Design review of the part built by this model. Coordinates are the model's own, in mm. Give positions to 0.01 mm unless a question says otherwise; leave off trailing zeros. Loops run counter-clockwise (first coordinate to the right, second up) from the corner with the lowest first, then second, coordinate; pieces in that order, holes last. Notation, with made-up numbers: M -19.75,-36.5 L 25.25,-36.5 A20 cw 25.25,-27.5 Z; hole C -30.5,83.25 d4. An arc over 180 degrees is marked long. Use a Markdown table: item, result. Add a question column.
(1) For probe 1 along Y at (x, z) = (40, 3.25); probe 2 along Y at (x, z) = (-7.75, 4.75); probe 3 along X at (y, z) = (13.5, 9), list the stretches that pass through material, from the lowest coordinate up.
(2) Add section A-A, the plane x = -40. Give the boundary of the cut face in (y, z).
(3) Insertion check: pin 1 Ø2.5 at (x, y) = (15.5, 0) entering from +Z. The pin has a flat end and moves straight along its axis. Give the tip position at first contact, or say it passes through.
(4) Draft analysis for pull direction Y (two halves, no side actions). For faces 1 (the face through (-43, 33, 6)), 2 (the face through (-1, 43, 6)), 3 (the face through (-1, -57, 6)), state which applies: pulls with the +Y half, pulls with the -Y half, needs draft (parallel to the pull), parting line crosses it, or undercut.
(5) Add section C-C, the plane x = -7.75. Give the boundary of the cut face in (y, z).
(6) Add section B-B, the plane y = -7. Give the boundary of the cut face in (x, z).
(7) Add section D-D, the plane z = 10. State how many separate pieces and enclosed holes the cut face has, then the cut area to 3 significant figures.
```python
from build123d import *

# Parameters (mm, degrees)
ESQUISSE1_R             = 18.5
BOSS_EXTRU_1_DEPTH      = 12
ESQUISSE2_R             = 2
ENL_V_MAT_EXTRU_1_DEPTH = 13
ESQUISSE3_R             = 6.25
ENL_V_MAT_EXTRU_2_DEPTH = 13
ESQUISSE4_W             = 100
ESQUISSE4_H             = 100
ESQUISSE4_R             = 18.5
BOSS_EXTRU_2_DEPTH      = 12
ESQUISSE5_R             = 3
ENL_V_MAT_EXTRU_3_DEPTH = 12


with BuildPart() as part:
    # Esquisse1 → Boss.-Extru.1 (new body)
    with BuildSketch(Plane.XY):
        Circle(ESQUISSE1_R)
    extrude(amount=BOSS_EXTRU_1_DEPTH)

    # Esquisse2 → Enlèv. mat.-Extru.1 (cut, through all)
    with BuildSketch(Plane.XY.offset(12)):
        with Locations((15.5, 0)):
            Circle(ESQUISSE2_R)
        with Locations((7.75, -13.423393759)):
            Circle(ESQUISSE2_R)
        with Locations((-7.75, -13.423393759)):
            Circle(ESQUISSE2_R)
        with Locations((-15.5, 0)):
            Circle(ESQUISSE2_R)
        with Locations((-7.75, 13.423393759)):
            Circle(ESQUISSE2_R)
        with Locations((7.75, 13.423393759)):
            Circle(ESQUISSE2_R)
    extrude(amount=-ENL_V_MAT_EXTRU_1_DEPTH, mode=Mode.SUBTRACT)

    # Esquisse3 → Enlèv. mat.-Extru.2 (cut, through all)
    with BuildSketch(Plane.XY.offset(12)):
        with Locations((0, -7)):
            Circle(ESQUISSE3_R)
    extrude(amount=-ENL_V_MAT_EXTRU_2_DEPTH, mode=Mode.SUBTRACT)

    # Esquisse4 → Boss.-Extru.2 (add)
    with BuildSketch(Plane.XY.offset(12)):
        with Locations((0, -7)):
            Rectangle(ESQUISSE4_W, ESQUISSE4_H)
        Circle(ESQUISSE4_R, mode=Mode.SUBTRACT)
    extrude(amount=-BOSS_EXTRU_2_DEPTH)

    # Esquisse5 → Enlèv. mat.-Extru.3 (cut)
    with BuildSketch(Plane.XY.offset(12)):
        with Locations((-40, 33)):
            Circle(ESQUISSE5_R)
        with Locations((40, 33)):
            Circle(ESQUISSE5_R)
        with Locations((40, -47)):
            Circle(ESQUISSE5_R)
        with Locations((-40, -47)):
            Circle(ESQUISSE5_R)
    extrude(amount=-ENL_V_MAT_EXTRU_3_DEPTH, mode=Mode.SUBTRACT)


solid = part.part
```
Established:
| question | item | result |
|---|---|---|
| 1 | probe 1 | -57 to -50, -44 to 30, 36 to 43 |
| 1 | probe 2 | -57 to -15.42, -11.42 to 11.42, 15.42 to 43 |
| 1 | probe 3 | -50 to -9.75, -5.75 to 5.75, 9.75 to 50 |
| 2 | outline | M -57,0 L -50,0 L -50,12 L -57,12 Z; M -44,0 L 30,0 L 30,12 L -44,12 Z; M 36,0 L 43,0 L 43,12 L 36,12 Z |
| 3 | pin 1 | through |
| 4 | face 1 | undercut |
| 4 | face 2 | pulls with the +Y half |
| 4 | face 3 | pulls with the -Y half |
| 5 | outline | M -57,0 L -15.42,0 L -15.42,12 L -57,12 Z; M -11.42,0 L 11.42,0 L 11.42,12 L -11.42,12 Z; M 15.42,0 L 43,0 L 43,12 L 15.42,12 Z |
| 6 | outline | M -50,0 L -6.25,0 L -6.25,12 L -50,12 Z; M 6.25,0 L 50,0 L 50,12 L 6.25,12 Z |
| 7 | separate pieces | 1 |
| 7 | enclosed holes | 11 |
| 7 | area | 9,690 mm^2 |
